The listing builds one solid part. Answer for the finished solid, in the listing's coordinates (mm). Give positions to 0.01 mm unless a question says otherwise; leave off trailing zeros. Write each loop counter-clockwise with the first axis right and the second up, starting at its lowest first coordinate (ties: lowest second). Pieces come first, ordered by that corner, then holes. Notation, with made-up numbers: (77.5, 14.25) - (132.5, 14.25) arc R21 ccw to (132.5, 24.25) - close; hole circle Ø1 at (-10.75, 45). An arc over 180 degrees is marked (long way). Write each question's results on one line, items separated by ' | '. Start each with the question number.
Q1. Section C-C (x = -246.5) is taken. Determine the outline of the cut face in (y, z).
Q2. Flat-ended cylindrical pins translate along their axes: pin 1 Ø3.5 at (x, z) = (-135, -2) entering from -Y; pin 2 Ø8 at (x, y) = (-152.5, -83.5) entering from -Z; pin 3 Ø1.6 at (y, z) = (161.5, -1.5) entering from -X; pin 4 Ø3.5 at (y, z) = (152.5, -1.5) entering from +X. Find the tip coordinate at first contact, or state that the pin passes through.
Q3. Find the intervals of material crossed by probe 1 along Z at (x, y) = (156, 60); probe 2 along Y at (x, z) = (-299.5, 3.25); probe 3 along X at (y, z) = (-143.5, 5.5), in increasing order.
Q4. Section A-A (y = 151) is taken. Determine the outline of the cut face in (x, z) (3 decimals).
Q5. Section B-B (x = 247.5) is taken. Determine the outline of the cut face in (y, z) (3 decimals).
Q6. Section D-D (y = 107) is taken. Determine the outline of the cut face in (x, z), plus the area to 3 significant figures.
```python
from build123d import *

# Parameters (mm, degrees)
F0_W     = 698.5
F0_H     = 355.6
F1_DEPTH = 25.4
F3_DEPTH = 25.401
F4_W     = 88.9
F4_H     = 44.45
F5_DEPTH = 3.175


with BuildPart() as f1:
    # F0 (on Top) → F1 (new body)
    with BuildSketch(Plane.XY):
        Rectangle(F0_W, F0_H)
    extrude(amount=F1_DEPTH)

    # F2 (on face) → F3 (cut, through all)
    with BuildSketch(Plane.XY.offset(25.4)):
        Polygon((-254, -177.8), (-349.25, -114.3), (-349.25, -177.8), align=None)
    extrude(amount=-F3_DEPTH, mode=Mode.SUBTRACT)

    # F4 (on face) → F5 (join)
    with BuildSketch(Plane(origin=(0, 0, 0), x_dir=(1, 0, 0), z_dir=(0, 0, -1))):
        with Locations((254, -155.575)):
            Rectangle(F4_W, F4_H)
        with Locations((-152.4, -155.575)):
            Rectangle(F4_W, F4_H)
    extrude(amount=F5_DEPTH)


solid = f1.part
```
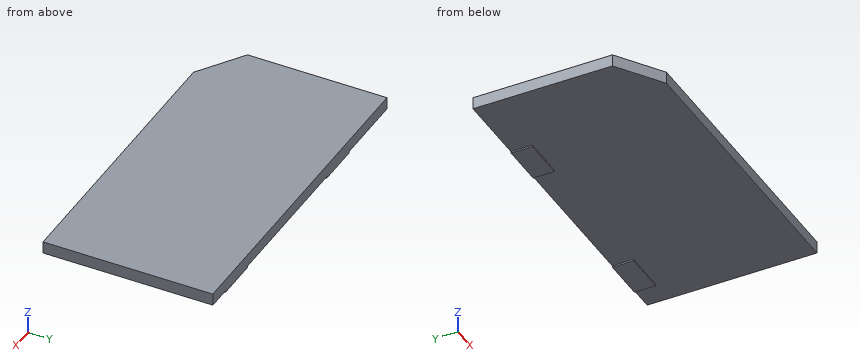
Answers below:
1) outline: (-177.8, 0) - (177.8, 0) - (177.8, 25.4) - (-177.8, 25.4) - close
2) pin 1: stops at y = 133.35 | pin 2: stops at z = 0 | pin 3: stops at x = -196.85 | pin 4: stops at x = 349.25
3) probe 1: z = 0 to 25.4 | probe 2: y = -147.47 to 177.8 | probe 3: x = -305.45 to 349.25
4) outline: (-349.25, 0) - (-196.85, 0) - (-196.85, -3.175) - (-107.95, -3.175) - (-107.95, 0) - (209.55, 0) - (209.55, -3.175) - (298.45, -3.175) - (298.45, 0) - (349.25, 0) - (349.25, 25.4) - (-349.25, 25.4) - close
5) outline: (-177.8, 0) - (133.35, 0) - (133.35, -3.175) - (177.8, -3.175) - (177.8, 25.4) - (-177.8, 25.4) - close
6) outline: (-349.25, 0) - (349.25, 0) - (349.25, 25.4) - (-349.25, 25.4) - close | area: 17,700 mm2
